```python
from build123d import *

# Parameters (mm, degrees)
SKETCH1_W           = 50
SKETCH1_H           = 50
BOSS_EXTRUDE1_DEPTH = 4
SKETCH2_R           = 2.874998181
CUT_EXTRUDE1_DEPTH  = 4
SKETCH3_W           = 50
SKETCH3_H           = 6.348267119
BOSS_EXTRUDE2_DEPTH = 4


with BuildPart() as part:
    # Sketch1 → Boss-Extrude1 (new body)
    with BuildSketch(Plane.XY):
        with Locations((25, 25)):
            Rectangle(SKETCH1_W, SKETCH1_H)
    extrude(amount=BOSS_EXTRUDE1_DEPTH)

    # Sketch2 → Cut-Extrude1 (cut)
    with BuildSketch(Plane.XY.offset(4)):
        with Locations((9.410896039, 40.009779151)):
            Circle(SKETCH2_R)
        with Locations((17.410896039, 40.009779151)):
            Circle(SKETCH2_R)
        with Locations((25.410896039, 40.009779151)):
            Circle(SKETCH2_R)
        with Locations((33.410896039, 40.009779151)):
            Circle(SKETCH2_R)
        with Locations((41.410896039, 40.009779151)):
            Circle(SKETCH2_R)
        with Locations((17.410896039, 30.009779151)):
            Circle(SKETCH2_R)
        with Locations((25.410896039, 30.009779151)):
            Circle(SKETCH2_R)
        with Locations((33.410896039, 30.009779151)):
            Circle(SKETCH2_R)
        with Locations((41.410896039, 30.009779151)):
            Circle(SKETCH2_R)
        with Locations((17.410896039, 20.009779151)):
            Circle(SKETCH2_R)
        with Locations((25.410896039, 20.009779151)):
            Circle(SKETCH2_R)
        with Locations((33.410896039, 20.009779151)):
            Circle(SKETCH2_R)
        with Locations((41.410896039, 20.009779151)):
            Circle(SKETCH2_R)
        with Locations((17.410896039, 10.009779151)):
            Circle(SKETCH2_R)
        with Locations((25.410896039, 10.009779151)):
            Circle(SKETCH2_R)
        with Locations((33.410896039, 10.009779151)):
            Circle(SKETCH2_R)
        with Locations((41.410896039, 10.009779151)):
            Circle(SKETCH2_R)
        with Locations((9.410896039, 30.009779151)):
            Circle(SKETCH2_R)
        with Locations((9.410896039, 20.009779151)):
            Circle(SKETCH2_R)
        with Locations((9.410896039, 10.009779151)):
            Circle(SKETCH2_R)
    extrude(amount=-CUT_EXTRUDE1_DEPTH, mode=Mode.SUBTRACT)

    # Sketch3 → Boss-Extrude2 (add)
    with BuildSketch(Plane(origin=(0, 0, 0), x_dir=(-1, 0, 0), z_dir=(0, 0, -1))):
        with Locations((-25, 46.825866441)):
            Rectangle(SKETCH3_W, SKETCH3_H)
    extrude(amount=BOSS_EXTRUDE2_DEPTH)


solid = part.part
```
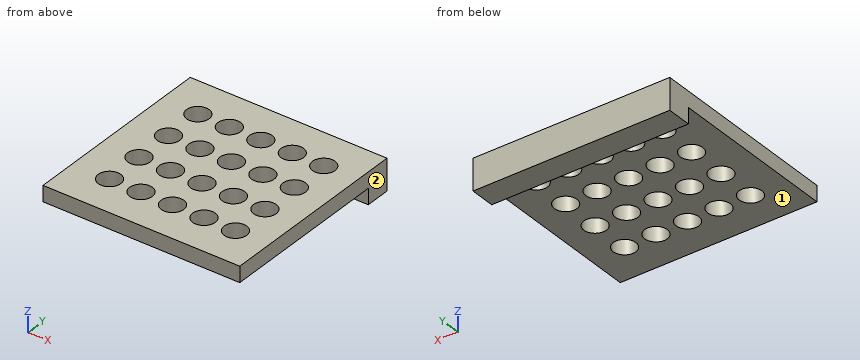
The model under review builds one solid part; all positions refer to its coordinate system, in mm. Face numbers are marked on the shaded views. A direction names the side the tool comes from. Round coordinates to 2 decimals unless told otherwise and drop trailing zeros. Order: outer loops, then holes, each group sorted by start corner. A loop starts at its lowest first (then second) coordinate and runs counter-clockwise, first axis right, second up. Notation, with made-up numbers: (30, 81) - (79, 81) arc R3 cw to (79, 86) - close; hole circle Ø11 at (18.5, 28.25). An arc over 180 degrees is marked (long way). Answer in a Markdown table with one row per item.
(1) For line 1 (X direction, y = 10, z = 0.5); line 2 (Y direction, x = 17.5, z = 2.25); line 3 (Y direction, x = 19, z = 1.5), list the stretches that pass through material, from the lowest coordinate up. Write a range as from..to.
Result set:
| item | result |
|---|---|
| line 1 | x = 0..6.54, 12.29..14.54, 20.29..22.54, 28.29..30.54, 36.29..38.54, 44.29..50 |
| line 2 | y = 0..7.14, 12.88..17.14, 22.88..27.14, 32.88..37.14, 42.88..50 |
| line 3 | y = 0..7.61, 12.41..17.61, 22.41..27.61, 32.41..37.61, 42.41..50 |
(2) Take a section at B-B on y = 32. Write out the cut boundary in (x, z), plus the area to 3 significant figures.
Result set:
| item | result |
|---|---|
| outline | (0, 0) - (7.34, 0) - (7.34, 4) - (0, 4) - close; (11.49, 0) - (15.34, 0) - (15.34, 4) - (11.49, 4) - close; (19.49, 0) - (23.34, 0) - (23.34, 4) - (19.49, 4) - close; (27.49, 0) - (31.34, 0) - (31.34, 4) - (27.49, 4) - close; (35.49, 0) - (39.34, 0) - (39.34, 4) - (35.49, 4) - close; (43.49, 0) - (50, 0) - (50, 4) - (43.49, 4) - close |
| area | 117 mm2 |
(3) Clearance check with a flat-ended pin moving along its axis: P1, Ø3, axis at x = 14.5, y = 18.5, coming from the -Z side. State where the tip first meets the part, or that it passes through.
Result set:
| item | result |
|---|---|
| P1 | stops at z = 0 |
(4) Take a section at C-C on z = 3.25. Count the separate pieces of the cut face and the enclosed holes in it, plus the area to 3 significant figures.
Result set:
| item | result |
|---|---|
| separate pieces | 1 |
| enclosed holes | 20 |
| area | 1,980 mm2 |
(5) Take a section at A-A on x = 16. Write out the cut boundary in (y, z).
Result set:
| item | result |
|---|---|
| outline | (0, 0) - (7.5, 0) - (7.5, 4) - (0, 4) - close; (12.51, 0) - (17.5, 0) - (17.5, 4) - (12.51, 4) - close; (22.51, 0) - (27.5, 0) - (27.5, 4) - (22.51, 4) - close; (32.51, 0) - (37.5, 0) - (37.5, 4) - (32.51, 4) - close; (42.51, 0) - (43.65, 0) - (43.65, -4) - (50, -4) - (50, 4) - (42.51, 4) - close |
(6) Machinability: for the marked faces 1 and 2, which of the approach directions +Z, -Z, +X, -X, +Y, -Y give a long, thin tool a straight path to every point of the face, cutting with its end or side? Answer none if there is none.
Result set:
| item | result |
|---|---|
| face 1 | -Z, +X, -X, -Y |
| face 2 | +Z, -Z, +X, +Y, -Y |
(7) Take a section at D-D on x = 29. Write out the cut boundary in (y, z), plus the area to 3 significant figures.
Result set:
| item | result |
|---|---|
| outline | (0, 0) - (43.65, 0) - (43.65, -4) - (50, -4) - (50, 4) - (0, 4) - close |
| area | 225 mm2 |
